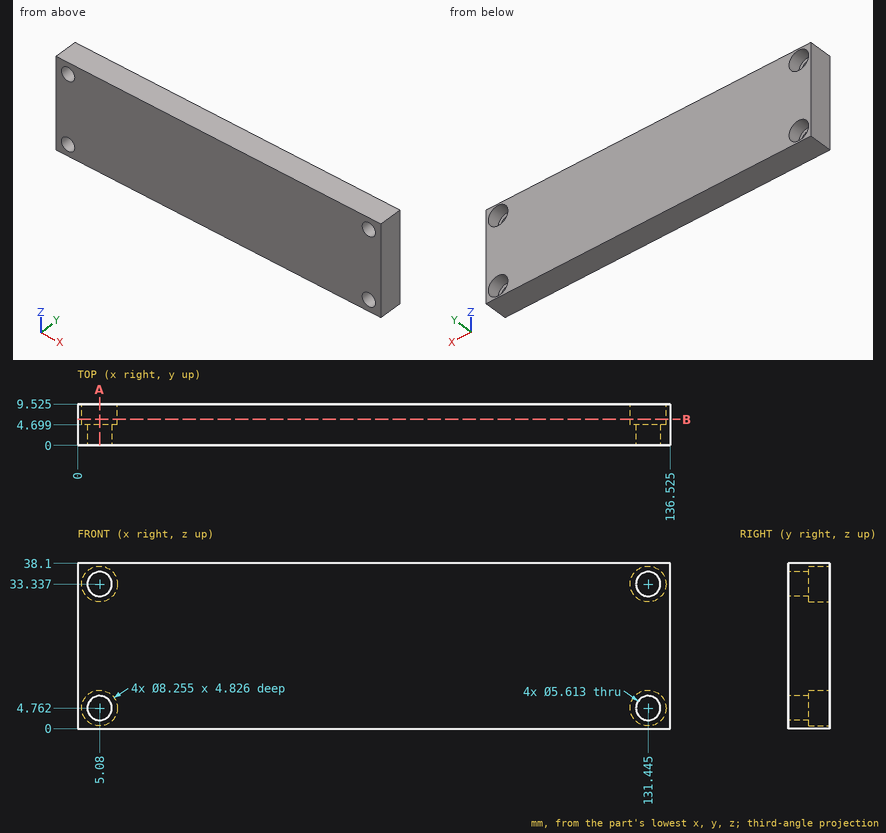
Study the drawing (mm; zero at the part's minimum x, y, z) and answer. Coordinates: 2 decimals unless noted, no trailing zeros. Loops run counter-clockwise (first coordinate to the right, second up) from the corner with the lowest first, then second, coordinate; pieces in that order, holes last. Notation, with made-up numbers: (39, -9.5) -> (59, -9.5) arc R23 ccw to (59, 25.5) -> close; hole circle Ø5 at (89, 30.5). An arc over 180 degrees is marked (long way). Write item = value, one per line. Start each with the question number.
1) The part is cut by section A-A, the plane x = 5.08. Determine the outline of the cut face in (y, z) (1 decimal).
2) The part is cut by section B-B, the plane y = 6. Determine the outline of the cut face in (x, z) (1 decimal), plus the area to 3 significant figures.
3) Given P1, Ø7.5, axis at x = 5.08, z = 33.34, coming from the -Y side, flat-ended and moving along its own axis, determine where the tip first touches the part or whether it passes through.
4) Find the intervals of material crossed by L1, parallel to X at y = 6.25, z = 4.5 (1 decimal); L2, parallel to Z at x = 5.08, y = 2.3 (1 decimal); L3, parallel to X at y = 5.25, z = 8 (1 decimal), in increasing order. Write a range as from..to.
Result:
q1.outline = (0, 0) -> (9.5, 0) -> (9.5, 0.6) -> (4.7, 0.6) -> (4.7, 2) -> (0, 2) -> close; (0, 7.6) -> (4.7, 7.6) -> (4.7, 8.9) -> (9.5, 8.9) -> (9.5, 29.2) -> (4.7, 29.2) -> (4.7, 30.5) -> (0, 30.5) -> close; (0, 36.1) -> (4.7, 36.1) -> (4.7, 37.5) -> (9.5, 37.5) -> (9.5, 38.1) -> (0, 38.1) -> close
q2.outline = (0, 0) -> (136.5, 0) -> (136.5, 38.1) -> (0, 38.1) -> close; hole circle Ø8.3 at (5.1, 4.8); hole circle Ø8.3 at (5.1, 33.3); hole circle Ø8.3 at (131.4, 4.8); hole circle Ø8.3 at (131.4, 33.3)
q2.area = 4,990 mm²
q3.P1 = 0
q4.L1 = 0..1, 9.2..127.3, 135.6..136.5
q4.L2 = 0..2, 7.6..30.5, 36.1..38.1
q4.L3 = 0..2.5, 7.6..128.9, 134..136.5
